Answer from the drawing. Dimensions are ordinates in mm from the lowest x, y and z of the part. Give positions to 0.01 mm unless a question says otherwise; leave off trailing zeros. Order: outer loops, then holes, each group sorted by start corner. A loop starts at its lowest first (then second) coordinate and runs counter-clockwise, first axis right, second up. Notation, with made-up numbers: (25.5, -25.5) - (51.5, -25.5) arc R20 cw to (51.5, 8.5) - close; hole circle Ø3 at (1.5, 48.25). An arc over 180 degrees is marked (long way). One line per item, written item: value. Start each with the question number.
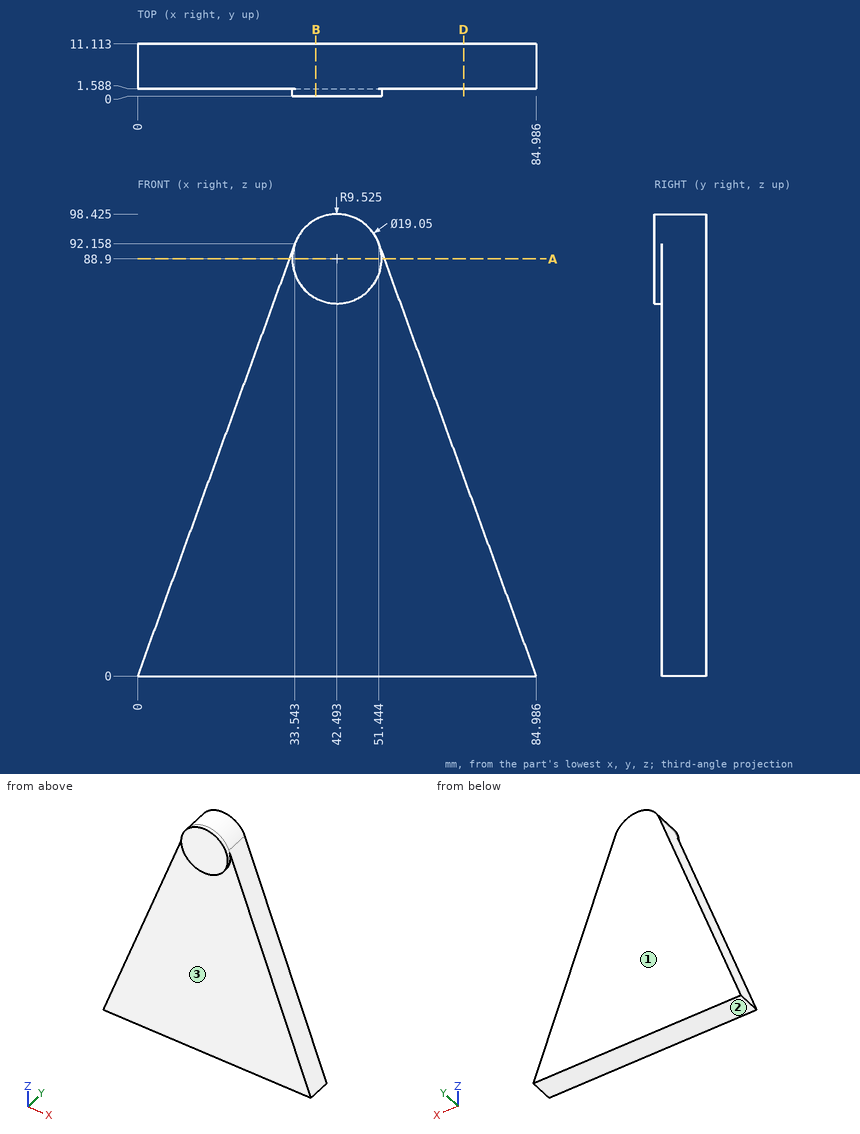
1) Find the intervals of material crossed by probe 1 along Y at (x, z) = (45, 50.5); probe 2 along X at (y, z) = (3, 40); probe 3 along Z at (x, y) = (36.5, 2.25) (1 decimal), in increasing order. Write a range as from..to.
2) Each of these flat-tipped pins is pushed along its axis until it touches: pin 1 (3 mm diameter, centred on x = 16, y = 6, fed in from -Z); pin 2 (1.5 mm diameter, centred on x = 55.5, z = 20, fed in from -Y); pin 3 (5 mm diameter, centred on x = 36.5, y = 9, fed in from +Z); pin 4 (4 mm diameter, centred on y = 4.5, z = 12, fed in from +X). Where does it stop, or does it pass through?
3) The mould has two halves that part along Y. Classify the marked faces 1, 2 and 3: +Y half, -Y half, draft (parallel to the pull), parting line (faces both ways), or undercut.
4) Section D-D on x = 69.5 is taken. Write down the section's boundary in (y, z).
5) Section B-B on x = 38 is taken. Write down the section's boundary in (y, z).
6) Section A-A on z = 88.9 is taken. Write down the section's boundary in (x, y).
Solved:
1. probe 1: y = 1.59..11.11
1. probe 2: x = 14.56..70.43
1. probe 3: z = 0..96.3
2. pin 1: stops at z = 0
2. pin 2: stops at y = 1.59
2. pin 3: stops at z = 97.76
2. pin 4: stops at x = 81.35
3. face 1: +Y half
3. face 2: draft
3. face 3: -Y half
4. outline: (1.59, 0) - (11.11, 0) - (11.11, 42.55) - (1.59, 42.55) - close
5. outline: (0, 80.5) - (1.59, 80.5) - (1.59, 0) - (11.11, 0) - (11.11, 97.3) - (0, 97.3) - close
6. outline: (32.36, 1.59) - (32.97, 1.59) - (32.97, 0) - (52.02, 0) - (52.02, 1.59) - (52.63, 1.59) - (52.63, 11.11) - (32.36, 11.11) - close
